```python
from build123d import *

# Parameters (mm, degrees)
CROQUIS1_W              = 78.5
CROQUIS1_H              = 75
SALIENTE_EXTRUIR1_DEPTH = 2
CROQUIS2_R              = 2.5
SALIENTE_EXTRUIR2_DEPTH = 4


with BuildPart() as part:
    # Croquis1 → Saliente-Extruir1 (new body)
    with BuildSketch(Plane(origin=(0, 0, 0), x_dir=(1, 0, 0), z_dir=(0, 1, 0))):
        Rectangle(CROQUIS1_W, CROQUIS1_H)
    extrude(amount=SALIENTE_EXTRUIR1_DEPTH)

    # Croquis2 → Saliente-Extruir2 (add)
    with BuildSketch(Plane(origin=(0, 2, 0), x_dir=(1, 0, 0), z_dir=(0, 1, 0))):
        with Locations(Location((0, 0, 0), (0, 0, 90))):
            Circle(CROQUIS2_R)
    extrude(amount=SALIENTE_EXTRUIR2_DEPTH)


solid = part.part
```
Design review of the part built by this model. Coordinates are the model's own, in mm. A direction names the side the tool comes from. Round coordinates to 2 decimals unless told otherwise and drop trailing zeros. Order: outer loops, then holes, each group sorted by start corner. A loop starts at its lowest first (then second) coordinate and runs counter-clockwise, first axis right, second up. Notation, with made-up numbers: M 44.25,-22 L 89.25,-22 A21 cw 89.25,-3 Z; hole C 5,47 d7. An arc over 180 degrees is marked long. Put each result on its own line as item: value.
Q1. Insertion check: pin 1 Ø2 at (x, z) = (7.5, 13.5) entering from +Y. The pin has a flat end and moves straight along its axis. Give the tip position at first contact, or say it passes through.
Reported:
pin 1: y = 2
Q2. Consider section C-C (y = 3.5). State the section outline as (x, z) points, and give its area (3 significant figures).
Reported:
outline: C 0,0 d5
area: 19.6 mm²
Q3. To check wall thickness, follow line 1 (Y direction, x = -20.5, z = 17.5). State the ranges of the line that lie inside material, in increasing order.
Reported:
line 1: 0 to 2
Q4. Consider section A-A (x = 0). State the section outline as (y, z) points.
Reported:
outline: M 0,-37.5 L 2,-37.5 L 2,-2.5 L 6,-2.5 L 6,2.5 L 2,2.5 L 2,37.5 L 0,37.5 Z
Q5. Consider section D-D (z = -21). State the section outline as (x, y) points.
Reported:
outline: M -39.25,0 L 39.25,0 L 39.25,2 L -39.25,2 Z
Q6. Machinability: for faces 1 (the face through (-1, 1, -37.5)), 2 (the face through (2.44, 3.97, 0.54)), which of the approach directions +Z, -Z, +X, -X, +Y, -Y give a long, thin tool a straight path to every point of the face, cutting with its end or side? Answer none if there is none.
Reported:
face 1: -Z, +X, -X, +Y, -Y
face 2: +Y
Q7. Consider section B-B (z = 0). State the section outline as (x, y) points, and give its area (3 significant figures).
Reported:
outline: M -39.25,0 L 39.25,0 L 39.25,2 L 2.5,2 L 2.5,6 L -2.5,6 L -2.5,2 L -39.25,2 Z
area: 177 mm²
